```python
from build123d import *

# Parameters (mm, degrees)
BOSS_EXTRU_1_OUTLINE_R   = 50
BOSS_EXTRU_1_OUTLINE_W   = 5
BOSS_EXTRU_1_OUTLINE_H   = 5
BOSS_EXTRU_1_OUTLINE_R_2 = 2.05
BOSS_EXTRU_1_OUTLINE_R_3 = 1.5
BOSS_EXTRU_1_DEPTH       = 5
SKETCH3_W                = 1
SKETCH3_H                = 8
CUT_EXTRUDE2_DEPTH       = 10


# Read off the part's stored shape, not the designer's step: Boss.-Extru.1
with BuildPart() as part:
    # Boss.-Extru.1 outline → Boss.-Extru.1 (new body)
    with BuildSketch(Plane.XY):
        Circle(BOSS_EXTRU_1_OUTLINE_R)
        Polygon((-37.262039705, -33.060254038), (-39.762039705, -28.730127019), (-35.431912686, -26.230127019), (-32.931912686, -30.560254038), align=None, mode=Mode.SUBTRACT)
        with Locations((-7.5, -46.3)):
            Rectangle(BOSS_EXTRU_1_OUTLINE_W, BOSS_EXTRU_1_OUTLINE_H, mode=Mode.SUBTRACT)
        with Locations((-16.666666667, -28.867513459)):
            Circle(BOSS_EXTRU_1_OUTLINE_R_2, mode=Mode.SUBTRACT)
        with Locations((-40.096976195, -23.15)):
            Circle(BOSS_EXTRU_1_OUTLINE_R_3, mode=Mode.SUBTRACT)
        Polygon((-42.931912686, -13.239745962), (-40.431912686, -17.569872981), (-44.762039705, -20.069872981), (-47.262039705, -15.739745962), align=None, mode=Mode.SUBTRACT)
        with Locations((-34.597845014, -19.975075132)):
            Circle(BOSS_EXTRU_1_OUTLINE_R_2, mode=Mode.SUBTRACT)
        with Locations((0, -46.3)):
            Circle(BOSS_EXTRU_1_OUTLINE_R_3, mode=Mode.SUBTRACT)
        with Locations((7.5, -46.3)):
            Rectangle(BOSS_EXTRU_1_OUTLINE_W, BOSS_EXTRU_1_OUTLINE_H, mode=Mode.SUBTRACT)
        with Locations((0, -39.950150265)):
            Circle(BOSS_EXTRU_1_OUTLINE_R_2, mode=Mode.SUBTRACT)
        with Locations((16.666666667, -28.867513459)):
            Circle(BOSS_EXTRU_1_OUTLINE_R_2, mode=Mode.SUBTRACT)
        Polygon((32.931912686, -30.560254038), (35.431912686, -26.230127019), (39.762039705, -28.730127019), (37.262039705, -33.060254038), align=None, mode=Mode.SUBTRACT)
        with Locations((34.597845014, -19.975075132)):
            Circle(BOSS_EXTRU_1_OUTLINE_R_2, mode=Mode.SUBTRACT)
        with Locations((40.096976195, -23.15)):
            Circle(BOSS_EXTRU_1_OUTLINE_R_3, mode=Mode.SUBTRACT)
        Polygon((47.262039705, -15.739745962), (44.762039705, -20.069872981), (40.431912686, -17.569872981), (42.931912686, -13.239745962), align=None, mode=Mode.SUBTRACT)
        with Locations((-33.333333333, 0)):
            Circle(BOSS_EXTRU_1_OUTLINE_R_2, mode=Mode.SUBTRACT)
        Polygon((-47.262039705, 15.739745962), (-44.762039705, 20.069872981), (-40.431912686, 17.569872981), (-42.931912686, 13.239745962), align=None, mode=Mode.SUBTRACT)
        with Locations((-40.096976195, 23.15)):
            Circle(BOSS_EXTRU_1_OUTLINE_R_3, mode=Mode.SUBTRACT)
        with Locations((-34.597845014, 19.975075132)):
            Circle(BOSS_EXTRU_1_OUTLINE_R_2, mode=Mode.SUBTRACT)
        with Locations((-16.671397032, 9.625235564)):
            Circle(BOSS_EXTRU_1_OUTLINE_R_2, mode=Mode.SUBTRACT)
        Polygon((-32.931912686, 30.560254038), (-35.431912686, 26.230127019), (-39.762039705, 28.730127019), (-37.262039705, 33.060254038), align=None, mode=Mode.SUBTRACT)
        with Locations((-16.666666667, 28.867513459)):
            Circle(BOSS_EXTRU_1_OUTLINE_R_2, mode=Mode.SUBTRACT)
        with Locations((-7.5, 46.3)):
            Rectangle(BOSS_EXTRU_1_OUTLINE_W, BOSS_EXTRU_1_OUTLINE_H, mode=Mode.SUBTRACT)
        Circle(BOSS_EXTRU_1_OUTLINE_R_2, mode=Mode.SUBTRACT)
        with Locations((33.333333333, 0)):
            Circle(BOSS_EXTRU_1_OUTLINE_R_2, mode=Mode.SUBTRACT)
        with Locations((34.597845014, 19.975075133)):
            Circle(BOSS_EXTRU_1_OUTLINE_R_2, mode=Mode.SUBTRACT)
        Polygon((42.931912686, 13.239745962), (40.431912686, 17.569872981), (44.762039705, 20.069872981), (47.262039705, 15.739745962), align=None, mode=Mode.SUBTRACT)
        with Locations((40.096976195, 23.15)):
            Circle(BOSS_EXTRU_1_OUTLINE_R_3, mode=Mode.SUBTRACT)
        with Locations((16.666666667, 28.867513459)):
            Circle(BOSS_EXTRU_1_OUTLINE_R_2, mode=Mode.SUBTRACT)
        with Locations((0, 39.950150265)):
            Circle(BOSS_EXTRU_1_OUTLINE_R_2, mode=Mode.SUBTRACT)
        with Locations((0, 46.3)):
            Circle(BOSS_EXTRU_1_OUTLINE_R_3, mode=Mode.SUBTRACT)
        with Locations((7.5, 46.3)):
            Rectangle(BOSS_EXTRU_1_OUTLINE_W, BOSS_EXTRU_1_OUTLINE_H, mode=Mode.SUBTRACT)
        Polygon((37.262039705, 33.060254038), (39.762039705, 28.730127019), (35.431912686, 26.230127019), (32.931912686, 30.560254038), align=None, mode=Mode.SUBTRACT)
    extrude(amount=BOSS_EXTRU_1_DEPTH)

    # Sketch3 → Cut-Extrude2 (cut)
    with BuildSketch(Plane.XY.offset(5)):
        with Locations((-10.5, 0)):
            Rectangle(SKETCH3_W, SKETCH3_H)
        with Locations((-22.833333333, 0)):
            Rectangle(SKETCH3_W, SKETCH3_H)
        Polygon((-13.233653965, 23.921361037), (-14.099679369, 23.421361037), (-12.349679369, 20.390272124), (-15.380768282, 18.640272124), (-14.880768282, 17.77424672), (-11.849679369, 19.52424672), (-10.099679369, 16.493157806), (-9.233653965, 16.993157806), (-10.983653965, 20.02424672), (-7.952565052, 21.77424672), (-8.452565052, 22.640272124), (-11.483653965, 20.890272124), align=None)
        Polygon((15.130768282, 18.207259422), (14.630768282, 17.341234018), (7.702565052, 21.341234018), (8.202565052, 22.207259422), align=None)
        Polygon((8.202565052, -22.207259422), (7.702565052, -21.341234018), (14.630768282, -17.341234018), (15.130768282, -18.207259422), align=None)
        Polygon((27.333333333, -0.5), (27.333333333, 0.5), (23.833333333, 0.5), (23.833333333, 4), (22.833333333, 4), (22.833333333, 0.5), (19.333333333, 0.5), (19.333333333, -0.5), (22.833333333, -0.5), (22.833333333, -4), (23.833333333, -4), (23.833333333, -0.5), align=None)
        Polygon((-14.099679369, -23.421361037), (-13.233653965, -23.921361037), (-11.483653965, -20.890272124), (-8.452565052, -22.640272124), (-7.952565052, -21.77424672), (-10.983653965, -20.02424672), (-9.233653965, -16.993157806), (-10.099679369, -16.493157806), (-11.849679369, -19.52424672), (-14.880768282, -17.77424672), (-15.380768282, -18.640272124), (-12.349679369, -20.390272124), align=None)
        Polygon((-20.834234776, 12.184801987), (-19.940304487, 11.668776346), (-20.102964744, 11.386925384), (-20.996895032, 11.902951025), (-21.517828526, 11.000607275), (-21.800380609, 11.163968654), (-21.279447115, 12.066312404), (-22.173377404, 12.582338045), (-22.010717147, 12.864189006), (-21.116786859, 12.348163365), (-20.596554487, 13.24840375), (-20.314002404, 13.085042371), align=None)
    extrude(amount=-CUT_EXTRUDE2_DEPTH, mode=Mode.SUBTRACT)


solid = part.part
```
Source: CAD feature listing. Evaluate the final solid. Frame: model axes, mm. Give positions to 0.01 mm unless a question says otherwise; leave off trailing zeros. Loops run counter-clockwise (first coordinate to the right, second up) from the corner with the lowest first, then second, coordinate; pieces in that order, holes last. Notation, with made-up numbers: (7, -34) - (56, -34) arc R26 ccw to (56, -14) - close; hole circle Ø4 at (-18.75, -33). An arc over 180 degrees is marked (long way). Use CSV: the item, a comma, the result in double quotes. Start each with the question number.
1. Pin query (flat end, axial travel): pin 1 (2 mm diameter, centred on y = 16, z = 4, fed in from +X); pin 2 (2 mm diameter, centred on x = -22.5, z = 1.5, fed in from -Y); pin 3 (1.8 mm diameter, centred on x = 40.1, y = -23.15, fed in from -Z); pin 4 (1.5 mm diameter, centred on y = 45.5, z = 3.5, fed in from +X). Return the tip coordinate at first contact, or that it passes through.
2. Ray query, L1, parallel to Y at x = 0, z = 2.85; L2, parallel to X at y = -3, z = 2.55; L3, parallel to Y at x = 5.5, z = 4.05. Return the intervals inside material, ascending.
3. Section D-D (y = 35.5). Output: boundary loops of the cut face in (x, z).
4. Section B-B (y = -46.3). Output: boundary loops of the cut face in (x, z).
5. Section C-C (z = 1.6). Count the separate pieces of the cut face and the enclosed holes in it, then the cut area to 3 significant figures.
6. Section A-A (x = 0). Output: boundary loops of the cut face in (y, z), then the cut area to 4 significant figures.
Response:
1,pin 1,"x = 47.7"
1,pin 2,"y = -45.14"
1,pin 3,"through"
1,pin 4,"x = 22.3"
2,L1,"-50 to -47.8, -44.8 to -42, -37.9 to -2.05, 2.05 to 37.9, 42 to 44.8, 47.8 to 50"
2,L2,"-49.91 to -23.33, -22.33 to -11, -10 to 22.83, 23.83 to 49.91"
2,L3,"-49.7 to -48.8, -43.8 to 43.8, 48.8 to 49.7"
3,outline,"(-35.21, 0) - (35.21, 0) - (35.21, 5) - (-35.21, 5) - close"
4,outline,"(-18.88, 0) - (-10, 0) - (-10, 5) - (-18.88, 5) - close; (-5, 0) - (-1.5, 0) - (-1.5, 5) - (-5, 5) - close; (1.5, 0) - (5, 0) - (5, 5) - (1.5, 5) - close; (10, 0) - (18.88, 0) - (18.88, 5) - (10, 5) - close"
5,separate pieces,"1"
5,enclosed holes,"40"
5,area,"7,250 mm²"
6,outline,"(-50, 0) - (-47.8, 0) - (-47.8, 5) - (-50, 5) - close; (-44.8, 0) - (-42, 0) - (-42, 5) - (-44.8, 5) - close; (-37.9, 0) - (-2.05, 0) - (-2.05, 5) - (-37.9, 5) - close; (2.05, 0) - (37.9, 0) - (37.9, 5) - (2.05, 5) - close; (42, 0) - (44.8, 0) - (44.8, 5) - (42, 5) - close; (47.8, 0) - (50, 0) - (50, 5) - (47.8, 5) - close"
6,area,"408.5 mm²"
